Geometry check sheet. Reference: the model listing, model coordinates, mm. A direction names the side the tool comes from. Coordinates: 2 decimals unless noted, no trailing zeros. Write each loop counter-clockwise with the first axis right and the second up, starting at its lowest first coordinate (ties: lowest second). Pieces come first, ordered by that corner, then holes. Notation, with made-up numbers: (68.25, 59) -> (82.25, 59) arc R31 cw to (82.25, 90) -> close; hole circle Ø5 at (53.25, 85.25). An arc over 180 degrees is marked (long way). Answer in a Markdown table with one row per item. Add a question column.
1. Set-up check for faces 1 (the flat face through (-42, -69, -5)), 2 (the flat face through (-21, -143, -5)), 3 (the cylindrical face through (-4.3, -5.4, -8.5)), 4 (the flat face through (-2, -88, -11.75)), 5 (the cylindrical face through (14.9, -176.8, -2.6)): record each of +Z, -Z, +X, -X, +Y, -Y from which the full face is reachable in a straight line by a thin tool's end or side.
2. Mould release check, pull along X, two halves, no side actions. Record for faces 6 (the flat face through (-21, -92, -10)), 7 (the flat face through (5, -170, -5)), 8 (the cylindrical face through (-36.219, -145.406, -4.93)), 9 (the flat face through (-47, -177, -5)): pulls with the +X half, pulls with the -X half, needs draft (parallel to the pull), parting line crosses it, or undercut.
3. Cross-section at A-A on z = -17. Record the cut outline in (x, y), and give its area (3 significant figures).
4. Cross-section at B-B on y = -180. Record the cut outline in (x, z), and give its area (3 significant figures).
5. Depth check by flat-ended pin: P1, Ø10, axis at y = -59.5, z = -8.5, coming from the +X side; P2, Ø4, axis at x = 12.05, z = -5, coming from the +Y side; P3, Ø6, axis at y = -94, z = -9.5, coming from the -X side; P4, Ø20, axis at y = -159, z = -12, coming from the -X side. Enter the tip coordinate at first touch or a pass-through.
6. Cross-section at C-C on y = -79. Record the cut outline in (x, z).
7. Cross-section at D-D on x = -19. Record the cut outline in (y, z).
8. Scan lines: L1, parallel to X at y = -183, z = -5; L2, parallel to X at y = -181.5, z = 7; L3, parallel to X at y = -16, z = -7. Record each from-to range of solid material in increasing order. Write a range as from..to.
```python
from build123d import *
from build123d.topology import SkipClean

# Parameters (mm, degrees)
SALIENTE_EXTRUIR1_DEPTH    = 10
SALIENTE_EXTRUIR2_DEPTH    = 10
SALIENTE_EXTRUIR3_DEPTH    = 10
SALIENTE_EXTRUIR4_DEPTH    = 1.75
SALIENTE_EXTRUIR5_START    = 1.75
SALIENTE_EXTRUIR5_DEPTH    = 1.75
CROQUIS26_W                = 5
CROQUIS26_H                = 35
SALIENTE_EXTRUIR6_DEPTH    = 1.75
CROQUIS27_W                = 5
CROQUIS27_H                = 35
SALIENTE_EXTRUIR7_DEPTH    = 11.75
CORTAR_EXTRUIR3_DEPTH      = 205.699932829
CORTAR_EXTRUIR3_DEPTH_BACK = 99.75
SALIENTE_EXTRUIR8_START    = -5
SALIENTE_EXTRUIR8_DEPTH    = 5
CROQUIS29_R                = 10
SALIENTE_EXTRUIR9_DEPTH    = 5
CORTAR_EXTRUIR5_DEPTH      = 206.22487666
CORTAR_EXTRUIR5_DEPTH_BACK = 206.22487666
SALIENTE_EXTRUIR11_START   = -8.5
CROQUIS32_R                = 20
SALIENTE_EXTRUIR11_DEPTH   = 8.5
CROQUIS33_R                = 20
SALIENTE_EXTRUIR12_DEPTH   = 8.5
CROQUIS34_R                = 5.05
CORTAR_EXTRUIR6_DEPTH      = 90
CROQUIS39_R                = 5.78
CORTAR_EXTRUIR7_DEPTH      = 1.5
CROQUIS40_R                = 4
SALIENTE_EXTRUIR13_DEPTH   = 20
CROQUIS41_R                = 1.5
CORTAR_EXTRUIR8_DEPTH      = 20


with BuildPart() as part:
    # Croquis1 → Saliente-Extruir1 (new body)
    with BuildSketch(Plane.XY):
        Polygon((0, -143), (0, -35), (-1.6, -35), (-37.4, -35), (-42, -35), (-42, -143), align=None)
    extrude(amount=-SALIENTE_EXTRUIR1_DEPTH)

    # Croquis3 → Saliente-Extruir2 (add)
    with BuildSketch(Plane.XY):
        with BuildLine():
            Line((-47, -141), (-47, -145))
            Line((-47, -145), (-47, -160))
            Line((-47, -160), (-47, -180))
            Line((-47, -180), (-47, -200))
            Line((-47, -200), (-38.5, -200))
            Line((-38.5, -200), (-38.5, -151))
            Line((-38.5, -151), (-38.5, -143))
            Line((-38.5, -143), (-42, -143))
            Line((-42, -143), (-42, -139))
            Line((-42, -139), (-45, -139))
            ThreePointArc((-45, -139), (-46.414213562, -139.585786438), (-47, -141))
        make_face()
        with BuildLine():
            Line((0, -143), (-11.5, -143))
            ThreePointArc((-11.5, -143), (-5.843145751, -145.343145751), (-3.5, -151))
            Line((-3.5, -151), (-3.5, -200))
            Line((-3.5, -200), (5, -200))
            Line((5, -200), (5, -143))
            Line((5, -143), (5, -141))
            ThreePointArc((5, -141), (4.414213562, -139.585786438), (3, -139))
            Line((3, -139), (0, -139))
            Line((0, -139), (0, -143))
        make_face()
    extrude(amount=-SALIENTE_EXTRUIR2_DEPTH)

    # Croquis21 → Saliente-Extruir3 (add)
    with BuildSketch(Plane.XY):
        with BuildLine():
            Line((-38.5, -143), (-38.5, -151))
            ThreePointArc((-38.5, -151), (-36.156854249, -145.343145751), (-30.5, -143))
            Line((-30.5, -143), (-38.5, -143))
        make_face()
    extrude(amount=-SALIENTE_EXTRUIR3_DEPTH)

    # Croquis22 → Saliente-Extruir4 (add)
    with BuildSketch(Plane(origin=(0, 0, -10), x_dir=(-1, 0, 0), z_dir=(0, 0, -1))):
        with BuildLine():
            Line((3.5, -200), (3.5, -156.87358131))
            Line((3.5, -156.87358131), (3.5, -151))
            Line((3.5, -151), (3.5, -141.333778868))
            ThreePointArc((3.5, -141.333778868), (3.709430585, -140.721406432), (4.25, -140.365533031))
            ThreePointArc((4.25, -140.365533031), (4.790569415, -140.00965963), (5, -139.397287194))
            Line((5, -139.397287194), (5, -35))
            Line((5, -35), (0, -35))
            Line((0, -35), (0, -139))
            Line((0, -139), (-3, -139))
            ThreePointArc((-3, -139), (-4.414213562, -139.585786438), (-5, -141))
            Line((-5, -141), (-5, -200))
            Line((-5, -200), (3.5, -200))
        make_face()
        with BuildLine():
            Line((42, -35), (37, -35))
            Line((37, -35), (37, -139.397287194))
            ThreePointArc((37, -139.397287194), (37.209430585, -140.00965963), (37.75, -140.365533031))
            ThreePointArc((37.75, -140.365533031), (38.290569415, -140.721406432), (38.5, -141.333778868))
            Line((38.5, -141.333778868), (38.5, -151))
            Line((38.5, -151), (38.5, -155.512462497))
            Line((38.5, -155.512462497), (38.5, -200))
            Line((38.5, -200), (47, -200))
            Line((47, -200), (47, -141))
            ThreePointArc((47, -141), (46.414213562, -139.585786438), (45, -139))
            Line((45, -139), (42, -139))
            Line((42, -139), (42, -35))
        make_face()
    extrude(amount=SALIENTE_EXTRUIR4_DEPTH)

    # Croquis24 → Saliente-Extruir5 (add)
    with BuildSketch(Plane.XY.offset(SALIENTE_EXTRUIR5_START)):
        with BuildLine():
            Line((-37, -141.498649254), (-37, -35))
            Line((-37, -35), (-42, -35))
            Line((-42, -35), (-42, -139))
            Line((-42, -139), (-45, -139))
            ThreePointArc((-45, -139), (-46.414213562, -139.585786438), (-47, -141))
            Line((-47, -141), (-47, -200))
            Line((-47, -200), (-38.5, -200))
            Line((-38.5, -200), (-38.5, -143.435140927))
            ThreePointArc((-38.5, -143.435140927), (-38.290569415, -142.822768491), (-37.75, -142.466895091))
            ThreePointArc((-37.75, -142.466895091), (-37.209430585, -142.11102169), (-37, -141.498649254))
        make_face()
        with BuildLine():
            Line((0, -35), (-5, -35))
            Line((-5, -35), (-5, -140.397287194))
            ThreePointArc((-5, -140.397287194), (-4.790569415, -141.00965963), (-4.25, -141.365533031))
            ThreePointArc((-4.25, -141.365533031), (-3.709430585, -141.721406432), (-3.5, -142.333778868))
            Line((-3.5, -142.333778868), (-3.5, -200))
            Line((-3.5, -200), (5, -200))
            Line((5, -200), (5, -141))
            ThreePointArc((5, -141), (4.414213562, -139.585786438), (3, -139))
            Line((3, -139), (0, -139))
            Line((0, -139), (0, -35))
        make_face()
    extrude(amount=-SALIENTE_EXTRUIR5_DEPTH)

    # Croquis26 → Saliente-Extruir6 (add)
    with BuildSketch(Plane.XY):
        with Locations((-39.5, -17.5)):
            Rectangle(CROQUIS26_W, CROQUIS26_H)
        with Locations((-2.5, -17.5)):
            Rectangle(CROQUIS26_W, CROQUIS26_H)
    extrude(amount=SALIENTE_EXTRUIR6_DEPTH)

    # Croquis27 → Saliente-Extruir7 (add)
    with BuildSketch(Plane(origin=(0, 0, 0), x_dir=(-1, 0, 0), z_dir=(0, 0, -1))):
        with Locations((2.5, -17.5)):
            Rectangle(CROQUIS27_W, CROQUIS27_H)
        with Locations((39.5, -17.5)):
            Rectangle(CROQUIS27_W, CROQUIS27_H)
    extrude(amount=SALIENTE_EXTRUIR7_DEPTH)

    # Croquis28 → Cortar-Extruir3 (cut, two sides: drawn at the far end of the back side and taken through both)
    with BuildSketch(Plane.ZY.offset(5).offset(-CORTAR_EXTRUIR3_DEPTH_BACK)):
        with BuildLine():
            ThreePointArc((-11.75, -2.621822718), (-8.62065099, -0.678471884), (-5, 0))
            Line((-5, 0), (-11.75, 0))
            Line((-11.75, 0), (-11.75, -2.621822718))
        make_face()
        with BuildLine():
            Line((1.75, -2.621822718), (1.75, 0))
            Line((1.75, 0), (-5, 0))
            ThreePointArc((-5, 0), (-1.37934901, -0.678471884), (1.75, -2.621822718))
        make_face()
    extrude(amount=CORTAR_EXTRUIR3_DEPTH + CORTAR_EXTRUIR3_DEPTH_BACK, mode=Mode.SUBTRACT)

    # Croquis28<5> → Saliente-Extruir8 (add)
    with BuildSketch(Plane.ZY.offset(5).offset(SALIENTE_EXTRUIR8_START)):
        with BuildLine():
            Line((-11.75, -17.378177282), (-11.75, -2.621822718))
            ThreePointArc((-11.75, -2.621822718), (-15, -10), (-11.75, -17.378177282))
        make_face()
        with BuildLine():
            ThreePointArc((5, -10), (4.151502609, -5.968871126), (1.75, -2.621822718))
            Line((1.75, -2.621822718), (1.75, -17.378177282))
            ThreePointArc((1.75, -17.378177282), (4.151502609, -14.031128874), (5, -10))
        make_face()
    extrude(amount=SALIENTE_EXTRUIR8_DEPTH)

    # Croquis29 → Saliente-Extruir9 (add)
    with BuildSketch(Plane(origin=(-37, 0, 0), x_dir=(0, 0, -1), z_dir=(1, 0, 0))):
        with Locations((5, -10)):
            Circle(CROQUIS29_R)
    extrude(amount=-SALIENTE_EXTRUIR9_DEPTH)

    # Croquis31 → Cortar-Extruir5 (cut, two sides: drawn at the far end of the back side and taken through both)
    with BuildSketch(Plane(origin=(-38.5, 0, 0), x_dir=(0, 0, -1), z_dir=(1, 0, 0)).offset(-CORTAR_EXTRUIR5_DEPTH_BACK)):
        with BuildLine():
            Line((-1.75, -200), (5, -200))
            ThreePointArc((5, -200), (1.574376792, -199.704443804), (-1.75, -198.826510564))
            Line((-1.75, -198.826510564), (-1.75, -200))
        make_face()
        with BuildLine():
            Line((11.75, -200), (11.75, -198.826510564))
            ThreePointArc((11.75, -198.826510564), (8.425623208, -199.704443804), (5, -200))
            Line((5, -200), (11.75, -200))
        make_face()
    extrude(amount=CORTAR_EXTRUIR5_DEPTH + CORTAR_EXTRUIR5_DEPTH_BACK, mode=Mode.SUBTRACT)

    # Croquis32 → Saliente-Extruir11 (add)
    with BuildSketch(Plane(origin=(-38.5, 0, 0), x_dir=(0, 0, -1), z_dir=(1, 0, 0)).offset(SALIENTE_EXTRUIR11_START)):
        with Locations((5, -180)):
            Circle(CROQUIS32_R)
    extrude(amount=SALIENTE_EXTRUIR11_DEPTH)

    # Croquis33 → Saliente-Extruir12 (add)
    with BuildSketch(Plane.ZY.offset(3.5)):
        with Locations((-5, -180)):
            Circle(CROQUIS33_R)
    extrude(amount=-SALIENTE_EXTRUIR12_DEPTH)

    # Croquis34 → Cortar-Extruir6 (cut)
    with BuildSketch(Plane.ZY.offset(42)):
        with Locations(Location((-5, -10, 0), (0, 0, 270))):
            Circle(CROQUIS34_R)
    extrude(amount=-CORTAR_EXTRUIR6_DEPTH, mode=Mode.SUBTRACT)

    # Croquis39 → Cortar-Extruir7 (cut)
    with SkipClean():  # the faces are left unmerged after this step: merging them gives an invalid solid
        with BuildSketch(Plane.ZY.offset(5)):
            with Locations(Location((-5, -10, 0), (0, 0, 270))):
                Circle(CROQUIS39_R)
        extrude(amount=-CORTAR_EXTRUIR7_DEPTH, mode=Mode.SUBTRACT)

    # Croquis40 → Saliente-Extruir13 (add)
    with SkipClean():  # the faces are left unmerged after this step: merging them gives an invalid solid
        with BuildSketch(Plane(origin=(5, 0, 0), x_dir=(0, 0, -1), z_dir=(1, 0, 0))):
            with Locations(Location((5, -180, 0), (0, 0, 270))):
                Circle(CROQUIS40_R)
            with BuildLine():
                Line((6.5, -182), (3.5, -182))
                ThreePointArc((3.5, -182), (5, -177.5), (6.5, -182))
            make_face(mode=Mode.SUBTRACT)
        extrude(amount=SALIENTE_EXTRUIR13_DEPTH)

    # Croquis41 → Cortar-Extruir8 (cut)
    with SkipClean():  # the faces are left unmerged after this step: merging them gives an invalid solid
        with BuildSketch(Plane(origin=(0, -182, 0), x_dir=(1, 0, 0), z_dir=(0, 1, 0))):
            with Locations(Location((18.048745385, 5, 0), (0, 0, 270))):
                Circle(CROQUIS41_R)
            with Locations(Location((12.048745385, 5, 0), (0, 0, 270))):
                Circle(CROQUIS41_R)
        extrude(amount=-CORTAR_EXTRUIR8_DEPTH, mode=Mode.SUBTRACT)


solid = part.part
```
Results found:
| question | item | result |
|---|---|---|
| 1 | face 1 | +Z, -Z, -X, +Y |
| 1 | face 2 | +Z, -Z, -Y |
| 1 | face 3 | none |
| 1 | face 4 | -Z, +X, -X |
| 1 | face 5 | +X |
| 2 | face 6 | undercut |
| 2 | face 7 | pulls with the +X half |
| 2 | face 8 | undercut |
| 2 | face 9 | pulls with the -X half |
| 3 | outline | (-47, -196) -> (-38.5, -196) -> (-38.5, -164) -> (-47, -164) -> close; (-3.5, -196) -> (5, -196) -> (5, -164) -> (-3.5, -164) -> close |
| 3 | area | 544 mm^2 |
| 4 | outline | (-47, -25) -> (-38.5, -25) -> (-38.5, 15) -> (-47, 15) -> close; (-3.5, -25) -> (5, -25) -> (5, -9) -> (25, -9) -> (25, -7.5) -> (5, -7.5) -> (5, -2.5) -> (25, -2.5) -> (25, -1) -> (5, -1) -> (5, 15) -> (-3.5, 15) -> close |
| 4 | area | 740 mm^2 |
| 5 | P1 | stops at x = 0 |
| 5 | P2 | stops at y = -176 |
| 5 | P3 | stops at x = -42 |
| 5 | P4 | stops at x = -47 |
| 6 | outline | (-42, -11.75) -> (-37, -11.75) -> (-37, -10) -> (-5, -10) -> (-5, -11.75) -> (0, -11.75) -> (0, 1.75) -> (-5, 1.75) -> (-5, 0) -> (-37, 0) -> (-37, 1.75) -> (-42, 1.75) -> close |
| 7 | outline | (-143, -10) -> (-35, -10) -> (-35, 0) -> (-143, 0) -> close |
| 8 | L1 | x = -47..-38.5, -3.5..10.55, 13.55..16.55, 19.55..25 |
| 8 | L2 | x = -47..-38.5, -3.5..5 |
| 8 | L3 | x = -42..-37, -5..0 |
